Model file for the job. Use its own axes, mm. A direction names the side the tool comes from. Coordinates: 2 decimals unless noted, no trailing zeros. Order: outer loops, then holes, each group sorted by start corner. A loop starts at its lowest first (then second) coordinate and runs counter-clockwise, first axis right, second up. Notation, with made-up numbers: M 9.25,57 L 24.25,57 A26 cw 24.25,89 Z; hole C -12.75,-8.75 d5. An arc over 180 degrees is marked long. Return JSON: item names as keys, results as strings.
```python
from build123d import *

# Parameters (mm, degrees)
F1_DEPTH = 3
F0_W     = 5
F0_H     = 12
F0_W_2   = 12
F0_H_2   = 5
F2_DEPTH = 13
F4_W     = 3.9998013438
F4_H     = 12
F4_W_2   = 12
F4_H_2   = 4
F5_DEPTH = 1.5


with BuildPart() as f1:
    # F0 (on Top) → F1 (new body)
    with BuildSketch(Plane.XY):
        Polygon((0, 7), (0, 12), (-12, 0), (-7, 0), (-7, -12), (12, -12), (12, 7), align=None)
        with BuildLine():
            ThreePointArc((-3.9597979746, 1.6970562748), (-3.9597979746, 3.9597979746), (-1.6970562748, 3.9597979746))
            Line((-1.6970562748, 3.9597979746), (7.4953318806, -5.2325901808))
            ThreePointArc((7.4953318806, -5.2325901808), (7.4953318806, -7.4953318806), (5.2325901808, -7.4953318806))
            Line((5.2325901808, -7.4953318806), (-3.9597979746, 1.6970562748))
        make_face(mode=Mode.SUBTRACT)
    extrude(amount=F1_DEPTH)

    # F0 (on Top) → F2 (join)
    with BuildSketch(Plane.XY):
        with Locations((-9.5, -6)):
            Rectangle(F0_W, F0_H)
        with Locations((6, 9.5)):
            Rectangle(F0_W_2, F0_H_2)
    extrude(amount=F2_DEPTH)

    # F4 (on offset) → F5 (join)
    with BuildSketch(Plane.XY.offset(13)):
        with Locations((-5.0000993281, -6)):
            Rectangle(F4_W, F4_H)
        with Locations((6, 5)):
            Rectangle(F4_W_2, F4_H_2)
    extrude(amount=-F5_DEPTH)


solid = f1.part
```
Item 1: Saw through at B-B (y = 1). Write the cut outline in (x, z).
Check result:
{"outline": "M -11,0 L -3.26,0 L -3.26,3 L -11,3 Z; M 1.26,0 L 12,0 L 12,3 L 1.26,3 Z"}
Item 2: Saw through at A-A (z = 12). Write the cut outline in (x, y), and give its area (3 significant figures).
Check result:
{"outline": "M -12,-12 L -3,-12 L -3,0 L -12,0 Z; M 0,3 L 12,3 L 12,12 L 0,12 Z", "area": "216 mm2"}
Item 3: Saw through at C-C (x = 6.75). Write the cut outline in (y, z), and give its area (3 significant figures).
Check result:
{"outline": "M -12,0 L -7.92,0 L -7.92,3 L -12,3 Z; M -4.49,0 L 12,0 L 12,13 L 3,13 L 3,11.5 L 7,11.5 L 7,3 L -4.49,3 Z", "area": "118 mm2"}
Item 4: Pull direction Z, two halves, no side cores. Call faces 5 (the flat face through (6, 8, 13)), 6 (the flat face through (6, 7, 7)), 7 (the flat face through (-6, -12, 2)): +Z half, -Z half, draft (parallel to the pull), parting line (faces both ways), or undercut.
Check result:
{"face 5": "+Z half", "face 6": "undercut", "face 7": "draft"}
Item 5: 3-axis set-ups, long thin cutter, end or side, ignore diameter. For faces 1 (the flat face through (0, 9, 8)), 2 (the flat face through (-5, -6, 11.5)), 3 (the flat face through (0.7, -2.96, 1.48)), 4 (the flat face through (-3, -6, 12)): which of +Z, -Z, +X, -X, +Y, -Y reach the whole face in a straight line?
Check result:
{"face 1": "+Z, -X, +Y, -Y", "face 2": "+X, +Y, -Y", "face 3": "+Z, -Z", "face 4": "+Z, +X, +Y, -Y"}
Item 6: Drop flat-ended pins along their axis: pin 1 Ø1.5 at (y, z) = (-5.5, 10) entering from +X; pin 2 Ø7 at (x, y) = (5.5, -1.5) entering from +Z; pin 3 Ø12 at (x, y) = (-5, 8) entering from -Z; pin 4 Ø7 at (x, z) = (-7, 7.5) entering from +Y. Give the stop position or say it passes through.
Check result:
{"pin 1": "stops at x = -7", "pin 2": "stops at z = 3", "pin 3": "stops at z = 0", "pin 4": "stops at y = 0"}
Item 7: Saw through at D-D (z = 1.5). Write the cut outline in (x, y).
Check result:
{"outline": "M -12,-12 L 12,-12 L 12,12 L 0,12 L -12,0 Z; hole M -3.96,1.7 L 5.23,-7.5 A1.6 ccw 7.5,-5.23 L -1.7,3.96 A1.6 ccw Z"}
Item 8: Wall check: line 1 (Z direction, x = -4.5, y = -3.25); line 2 (Z direction, x = 8.5, y = -5); line 3 (X direction, y = -7.5, z = 4). Give the ranges that are in metal, low to high.
Check result:
{"line 1": "z = 0 to 3, 11.5 to 13", "line 2": "z = 0 to 3", "line 3": "x = -12 to -7"}
